```python
from build123d import *

# Parameters (mm, degrees)
SKETCH2_R           = 40
BOSS_EXTRUDE1_DEPTH = 200
CUT_EXTRUDE1_START  = 200
SKETCH4_R           = 60
CUT_EXTRUDE1_DEPTH  = 100


with BuildPart() as part:
    # Sketch2 → Boss-Extrude1 (new body)
    with BuildSketch(Plane(origin=(0, 0, 0), x_dir=(0, 0, -1), z_dir=(1, 0, 0))):
        with BuildLine():
            ThreePointArc((1495.529247778, 67.272238992), (1475.827854944, 88.899495683), (1468.695495681, 117.272238992))
            Line((1468.695495681, 117.272238992), (788.695495681, 117.272238992))
            ThreePointArc((788.695495681, 117.272238992), (781.563136418, 88.899495683), (761.861743585, 67.272238992))
            Line((761.861743585, 67.272238992), (1495.529247778, 67.272238992))
        make_face()
        with BuildLine():
            Line((780.657019908, 147.272238992), (1476.733971454, 549.152454344))
            ThreePointArc((1476.733971454, 549.152454344), (1468.769326722, 582.128067523), (1479.961523957, 614.152454344))
            Line((1479.961523957, 614.152454344), (722.751592411, 176.977096532))
            ThreePointArc((722.751592411, 176.977096532), (756.081623557, 170.657630252), (780.657019908, 147.272238992))
        make_face()
        with BuildLine():
            ThreePointArc((1578.695495681, 545.98620644), (1557.068238991, 526.284813607), (1528.695495681, 519.152454344))
            Line((1528.695495681, 519.152454344), (1528.695495681, 177.272238992))
            ThreePointArc((1528.695495681, 177.272238992), (1557.068238991, 170.139879729), (1578.695495681, 150.438486896))
            Line((1578.695495681, 150.438486896), (1578.695495681, 545.98620644))
        make_face()
        with BuildLine():
            ThreePointArc((780.657019908, 147.272238992), (670.739946104, 101.743096286), (788.695495681, 117.272238992))
            ThreePointArc((788.695495681, 117.272238992), (786.651045259, 132.801381698), (780.657019908, 147.272238992))
        make_face()
        with Locations((728.695495681, 117.272238992)):
            Circle(SKETCH2_R, mode=Mode.SUBTRACT)
        with BuildLine():
            ThreePointArc((1468.695495681, 117.272238992), (1486.26908881, 159.698645863), (1528.695495681, 177.272238992))
            ThreePointArc((1528.695495681, 177.272238992), (1571.121902553, 74.845832121), (1468.695495681, 117.272238992))
        make_face()
        with Locations((1528.695495681, 117.272238992)):
            Circle(SKETCH2_R, mode=Mode.SUBTRACT)
        with BuildLine():
            ThreePointArc((1528.695495681, 519.152454344), (1558.695495681, 631.113978571), (1476.733971454, 549.152454344))
            ThreePointArc((1476.733971454, 549.152454344), (1498.695495681, 527.190930117), (1528.695495681, 519.152454344))
        make_face()
        with Locations((1528.695495681, 579.152454344)):
            Circle(SKETCH2_R, mode=Mode.SUBTRACT)
    extrude(amount=BOSS_EXTRUDE1_DEPTH)

    # Sketch4 → Cut-Extrude1 (cut)
    with BuildSketch(Plane(origin=(0, 0, 0), x_dir=(0, 0, -1), z_dir=(1, 0, 0)).offset(CUT_EXTRUDE1_START)):
        with Locations((728.695495681, 117.272238992)):
            Circle(SKETCH4_R)
    extrude(amount=-CUT_EXTRUDE1_DEPTH, mode=Mode.SUBTRACT)


solid = part.part
```
The listing builds one solid part. Answer for the finished solid, in the listing's coordinates (mm). A direction names the side the tool comes from. Give positions to 0.01 mm unless a question says otherwise; leave off trailing zeros. Loops run counter-clockwise (first coordinate to the right, second up) from the corner with the lowest first, then second, coordinate; pieces in that order, holes last. Notation, with made-up numbers: (-6.75, 29.5) - (35.25, 29.5) arc R18 ccw to (35.25, 39.5) - close; hole circle Ø2 at (-6, -28). An arc over 180 degrees is marked (long way). Return JSON: item names as keys, results as strings. Group by question number.
1. Find section B-B (z = -1518.5). Write down the section's boundary in (x, y).
2. Given pin 1 Ø5 at (x, z) = (59, -1391.5) entering from -Y; pin 2 Ø1 at (x, y) = (175, 485.5) entering from +Z; pin 3 Ø4 at (x, z) = (88.5, -1059) entering from +Y, each flat-ended and moving along its own axis, determine where each tip first touches the part or whether it passes through.
3. Find section D-D (z = -969.5). Write down the section's boundary in (x, y), then the cut area to 3 significant figures.
4. Find section C-C (x = 129.5). Write down the section's boundary in (y, z), then the cut area to 3 significant figures.
5. Determine the mould class of faces 1 (the cylindrical face through (98.6, 554.813, -1496.953)), 2 (the flat face through (98.6, 398.625, -1106.657)), 3 (the flat face through (100, 78, -741)), 4 (the cylindrical face through (98.6, 527.41, -1498.32)) for opening direction Z: pulls with the +Z half, pulls with the -Z half, needs draft (parallel to the pull), parting line crosses it, or undercut.
6. Straight lines are drawn through the part: line 1 (Y direction, x = 8, z = -1522.5); line 2 (Z direction, x = 86.5, y = 95.5); line 3 (Z direction, x = 145, y = 271). For each, find the intervals that lie inside material, in ascending order. Write a range as [from, to].
7. Find section A-A (y = 381.5). Write down the section's boundary in (x, z).
8. Which of the six approach directions +Z, -Z, +X, -X, +Y, -Y give full straight-line access (tool end or side, diameter ignored) to faces 5 (the cylindrical face through (150.7, 88.54, -781.37)), 6 (the flat face through (99, 345, -1578.695)), 7 (the cylindrical face through (98.6, 159.23, -1485.805))?
Verdict:
{
 "1": {"outline": "(0, 58.14) - (200, 58.14) - (200, 78.59) - (0, 78.59) - close; (0, 155.95) - (200, 155.95) - (200, 176.4) - (0, 176.4) - close; (0, 520.03) - (200, 520.03) - (200, 540.47) - (0, 540.47) - close; (0, 617.83) - (200, 617.83) - (200, 638.28) - (0, 638.28) - close"},
 "2": {"pin 1": "stops at y = 67.27", "pin 2": "stops at z = -1256.26", "pin 3": "stops at y = 372.26"},
 "3": {"outline": "(0, 67.27) - (200, 67.27) - (200, 117.27) - (0, 117.27) - close; (0, 256.3) - (200, 256.3) - (200, 319.44) - (0, 319.44) - close", "area": "22,600 mm^2"},
 "4": {"outline": "(67.27, -1495.53) arc R60 ccw to (150.44, -1578.7) - (545.99, -1578.7) arc R60 ccw to (614.15, -1479.96) - (176.98, -722.75) arc R60 cw to (147.27, -780.66) - (549.15, -1476.73) arc R60 ccw to (519.15, -1528.7) - (177.27, -1528.7) arc R60 ccw to (117.27, -1468.7) - (117.27, -788.7) arc R60 cw to (67.27, -761.86) - close; hole circle Ø80 at (117.27, -1528.7); hole circle Ø80 at (579.15, -1528.7)", "area": "110,000 mm^2"},
 "5": {"face 1": "undercut", "face 2": "pulls with the +Z half", "face 3": "needs draft", "face 4": "undercut"},
 "6": {"line 1": "y = [57.59, 77.75], [156.79, 176.95], [519.47, 539.64], [618.67, 638.83]", "line 2": "z = [-1584.61, -1562.25], [-1495.14, -762.25], [-695.14, -672.79]", "line 3": "z = [-1578.7, -1528.7], [-994.96, -885.6]"},
 "7": {"outline": "(0, -1578.7) - (200, -1578.7) - (200, -1528.7) - (0, -1528.7) - close; (0, -1186.35) - (200, -1186.35) - (200, -1077) - (0, -1077) - close"},
 "8": {"face 5": "+Z, +X", "face 6": "-Z, +X, -X", "face 7": "+X, -X"}
}
